Geometry: final body of the model. Coordinates: model frame, mm. Give positions to 0.01 mm unless a question says otherwise; leave off trailing zeros. Loops run counter-clockwise (first coordinate to the right, second up) from the corner with the lowest first, then second, coordinate; pieces in that order, holes last.
1. First-contact query: P1, Ø1.5, axis at x = -40, z = 0.5, coming from the +Y side. Flat tip, straight axial feed; report the tip coordinate or a pass-through.
2. Section B-B, the plane x = -70. Output: boundary loops of the cut face in (y, z), then the cut area to 3 significant figures.
3. Section C-C, the plane y = 95.5. Output: boundary loops of the cut face in (x, z), then the cut area to 3 significant figures.
4. Material intervals for line 1 along Y through (x, z) = (-110.5, 2.6); line 2 along Y through (x, z) = (-47, 1.5); line 3 along X through (y, z) = (73, 0.6), sorted ascending.
5. Section A-A, the plane z = 2.05. Output: boundary loops of the cut face in (x, y), then the cut area to 3 significant figures.
6. Draft query along X for faces 1 (the face through (36.98, 66.31, 1.48)), 2 (the face through (-73.01, -24.79, 1.48)), 3 (the face through (9.233, -9.331, 1.479)), 4 (the face through (-4, 5, 0)). Return one class per face: +X half, -X half, draft (parallel to the pull), parting line (faces both ways), or undercut.
Autodesk Inventor part; units mm, degrees
ref_plane "YZ Plane" through (0, 0, 0) normal (1, 0, 0) x (0, 1, 0)
ref_plane "XZ Plane" through (0, 0, 0) normal (0, 1, 0) x (-1, 0, 0)
ref_plane "XY Plane" through (0, 0, 0) normal (0, 0, 1) x (1, 0, 0)
sketch "草圖1" plane through (0, 0, 0) normal (0, 0, 1) x (1, 0, 0)
  arc A0 (-17.0574, -3.0077) -> (5.924, 16.276) centre (-22.2668, 26.5366) ccw
  line L0 (5.924, 16.276) -> (41.0424, 112.7631)
  line L1 (-118.1769, -20.8378) -> (-17.0574, -3.0077)
  line L2 (-118.1769, -20.8378) -> (-26.5575, -28.8534)
  arc A1 (-26.5575, -28.8534) -> (33.0268, 21.1437) centre (-21.764, 25.9373) ccw
  line L3 (33.0268, 21.1437) -> (41.0424, 112.7631)
  circle A2 centre (7.3253, -8.7299) radius 2
  arc A3 (-17.5783, -0.0533) -> (3.1049, 17.302) centre (-22.2668, 26.5366) ccw
  line L4 (3.1049, 17.302) -> (46.017, 135.2022)
  line L5 (46.017, 135.2022) -> (36.0153, 20.8822)
  arc A4 (-26.819, -31.842) -> (36.0153, 20.8822) centre (-21.764, 25.9373) ccw
  line L6 (-26.819, -31.842) -> (-141.1389, -21.8403)
  line L7 (-141.1389, -21.8403) -> (-17.5783, -0.0533)
  line L8 (41.0424, 112.7631) -> (37.9484, 113.0338)
  line L9 (-118.1769, -20.8378) -> (-117.9062, -17.7438)
  point P0 (0, 0)
  dimension "d0" = 55
  dimension "d1" = 4
  dimension "d2" = 23
  dimension "d3" = 23
  dimension "d6" = 3
extrude "擠出1" add sketch "草圖1" along normal blind 3 contours L1 L9 L7 A3 L4 L8 L0 A0 | A0 L0 L3 A1 L2 L1
sketch "草圖2" plane through (0, 0, 3) normal (0, 0, 1) x (1, 0, 0)
  arc A0 (-26.5575, -28.8534) -> (33.0268, 21.1437) centre (-21.764, 25.9373) ccw
  line L0 (33.0268, 21.1437) -> (41.0424, 112.7631)
  line L1 (41.0424, 112.7631) -> (37.9484, 113.0338)
  line L2 (37.9484, 113.0338) -> (3.1049, 17.302)
  arc A1 (-17.5783, -0.0533) -> (3.1049, 17.302) centre (-22.2668, 26.5366) ccw
  line L3 (-17.5783, -0.0533) -> (-117.9062, -17.7438)
  line L4 (-117.9062, -17.7438) -> (-118.1769, -20.8378)
  line L5 (-118.1769, -20.8378) -> (-26.5575, -28.8534)
  circle A2 centre (7.3253, -8.7299) radius 2
  point P0 (0, 0)
equation "\"d3\" = d2"
properties part number "sus_2"
Answers below:
1. P1: stops at y = -3.87
2. outline: (-25.05, 0) - (-9.3, 0) - (-9.3, 3) - (-25.05, 3) - close
2. area: 47.3 mm2
3. outline: (31.57, 0) - (39.53, 0) - (39.53, 3) - (31.57, 3) - close
3. area: 23.9 mm2
4. line 1: y = -21.51 to -16.44
4. line 2: y = -27.06 to -5.24
4. line 3: x = 23.38 to 37.56
5. outline: (-118.18, -20.84) - (-26.56, -28.85) arc R55 ccw to (33.03, 21.14) - (41.04, 112.76) - (37.95, 113.03) - (3.1, 17.3) arc R27 cw to (-17.58, -0.05) - (-117.91, -17.74) - close; hole circle Ø4 at (7.33, -8.73)
5. area: 4,650 mm2
6. face 1: +X half
6. face 2: -X half
6. face 3: undercut
6. face 4: draft
